Input: part model. Units: mm. Frame: model coordinates. A direction names the side the tool comes from. Round coordinates to 2 decimals unless told otherwise and drop trailing zeros. Write each loop counter-clockwise with the first axis right and the second up, starting at its lowest first coordinate (ties: lowest second). Pieces come first, ordered by that corner, then holes. Notation, with made-up numbers: (42, 75) - (50, 75) arc R23 cw to (50, 87) - close; hole circle Ø10 at (50.5, 67). An arc over 180 degrees is marked (long way). Use one line per item in the form item = value.
```python
from build123d import *

# Parameters (mm, degrees)
BOSS_EXTRUDE1_DEPTH   = 150
BOSS_EXTRUDE2_DEPTH   = 150
BOSS_EXTRUDE2_2_DEPTH = 150
SKETCH3_W             = 750
SKETCH3_H             = 15
BOSS_EXTRUDE3_DEPTH   = 150


with BuildPart() as part:
    # Sketch1 → Boss-Extrude1 (new body)
    with BuildSketch(Plane.XY):
        Polygon((0, 640), (540, 640), (540, 0), (525, 0), (525, 220), (495, 220), (495, 235), (525, 235), (525, 355), (495, 355), (495, 370), (525, 370), (525, 490), (495, 490), (495, 505), (525, 505), (525, 625), (365, 625), (365, 505), (395, 505), (395, 490), (365, 490), (365, 370), (395, 370), (395, 355), (365, 355), (365, 235), (395, 235), (395, 220), (365, 220), (365, 0), (350, 0), (350, 220), (320, 220), (320, 235), (350, 235), (350, 355), (320, 355), (320, 370), (350, 370), (350, 490), (320, 490), (320, 505), (350, 505), (350, 625), (190, 625), (190, 505), (220, 505), (220, 490), (190, 490), (190, 370), (220, 370), (220, 355), (190, 355), (190, 235), (220, 235), (220, 220), (190, 220), (190, 0), (175, 0), (175, 220), (145, 220), (145, 235), (175, 235), (175, 355), (145, 355), (145, 370), (175, 370), (175, 490), (145, 490), (145, 505), (175, 505), (175, 625), (15, 625), (15, 505), (45, 505), (45, 490), (15, 490), (15, 370), (45, 370), (45, 355), (15, 355), (15, 235), (45, 235), (45, 220), (15, 220), (15, 0), (0, 0), align=None)
    extrude(amount=BOSS_EXTRUDE1_DEPTH)



with BuildPart() as body_2:
    # Sketch2 → Boss-Extrude2 (new body)
    with BuildSketch(Plane.XY):
        Polygon((560, 235), (605, 235), (605, 220), (575, 220), (575, 0), (560, 0), align=None)
    extrude(amount=BOSS_EXTRUDE2_DEPTH)


with BuildPart() as body_3:
    # Sketch2 → Boss-Extrude2 2 (new body)
    with BuildSketch(Plane.XY):
        Polygon((735, 0), (735, 220), (705, 220), (705, 235), (750, 235), (750, 0), align=None)
    extrude(amount=BOSS_EXTRUDE2_2_DEPTH)


with BuildPart() as part_1:
    add(part.part)

    add(body_2.part)  # Boss-Extrude3 merges body 2

    add(body_3.part)  # Boss-Extrude3 merges body 3
    # Sketch3 → Boss-Extrude3 (add)
    with BuildSketch(Plane.XY.offset(150)):
        with Locations((375, -7.5)):
            Rectangle(SKETCH3_W, SKETCH3_H)
    extrude(amount=-BOSS_EXTRUDE3_DEPTH)


solid = part_1.part
```
(1) Draft query along X for faces 3 (the face through (30, 370, 74)), 4 (the face through (750, 108, 76)), 5 (the face through (370, -15, 76)), 6 (the face through (335, 505, 74)). Return one class per face: released by +X, released by -X, zero draft, split by the parting line, or undercut.
Derived:
face_3 = undercut
face_4 = released by +X
face_5 = zero draft
face_6 = undercut
(2) Access query for faces 1 (the face through (720, 220, 74)), 2 (the face through (0, 308, 76)). Directions: +Z, -Z, +X, -X, +Y, -Y. A direction counts if a zero-diameter tool reaches every point of the face in a straight line with its end or side. Return the directions, or none.
Derived:
face_1 = +Z, -Z
face_2 = +Z, -Z, -X, +Y, -Y
(3) Cut plane C-C on y = 544. Output: boundary loops of the cut face in (x, z), then the cut area to 3 significant figures.
Derived:
outline = (0, 0) - (15, 0) - (15, 150) - (0, 150) - close; (175, 0) - (190, 0) - (190, 150) - (175, 150) - close; (350, 0) - (365, 0) - (365, 150) - (350, 150) - close; (525, 0) - (540, 0) - (540, 150) - (525, 150) - close
area = 9,000 mm^2
(4) Cut plane B-B on x = 299.5. Output: boundary loops of the cut face in (y, z).
Derived:
outline = (-15, 0) - (0, 0) - (0, 150) - (-15, 150) - close; (625, 0) - (640, 0) - (640, 150) - (625, 150) - close
(5) Cut plane A-A on y = 148. Output: boundary loops of the cut face in (x, z).
Derived:
outline = (0, 0) - (15, 0) - (15, 150) - (0, 150) - close; (175, 0) - (190, 0) - (190, 150) - (175, 150) - close; (350, 0) - (365, 0) - (365, 150) - (350, 150) - close; (525, 0) - (540, 0) - (540, 150) - (525, 150) - close; (560, 0) - (575, 0) - (575, 150) - (560, 150) - close; (735, 0) - (750, 0) - (750, 150) - (735, 150) - close
(6) Material intervals for L1, parallel to X at y = 596, z = 83; L2, parallel to X at y = 20, z = 91; L3, parallel to X at y = 227, z = 48, sorted ascending.
Derived:
L1 = 0 to 15, 175 to 190, 350 to 365, 525 to 540
L2 = 0 to 15, 175 to 190, 350 to 365, 525 to 540, 560 to 575, 735 to 750
L3 = 0 to 45, 145 to 220, 320 to 395, 495 to 540, 560 to 605, 705 to 750
(7) Cut plane D-D on z = 88. Count the separate pieces of the cut face and the enclosed holes in it, then the cut area to 3 significant figures.
Derived:
separate_pieces = 1
enclosed_holes = 3
area = 72,900 mm^2
